Here's the drawing with two shaded views (mm, measured from the low corner). I have some questions. Give positions to 0.01 mm unless a question says otherwise; leave off trailing zeros. Loops run counter-clockwise (first coordinate to the right, second up) from the corner with the lowest first, then second, coordinate; pieces in that order, holes last.
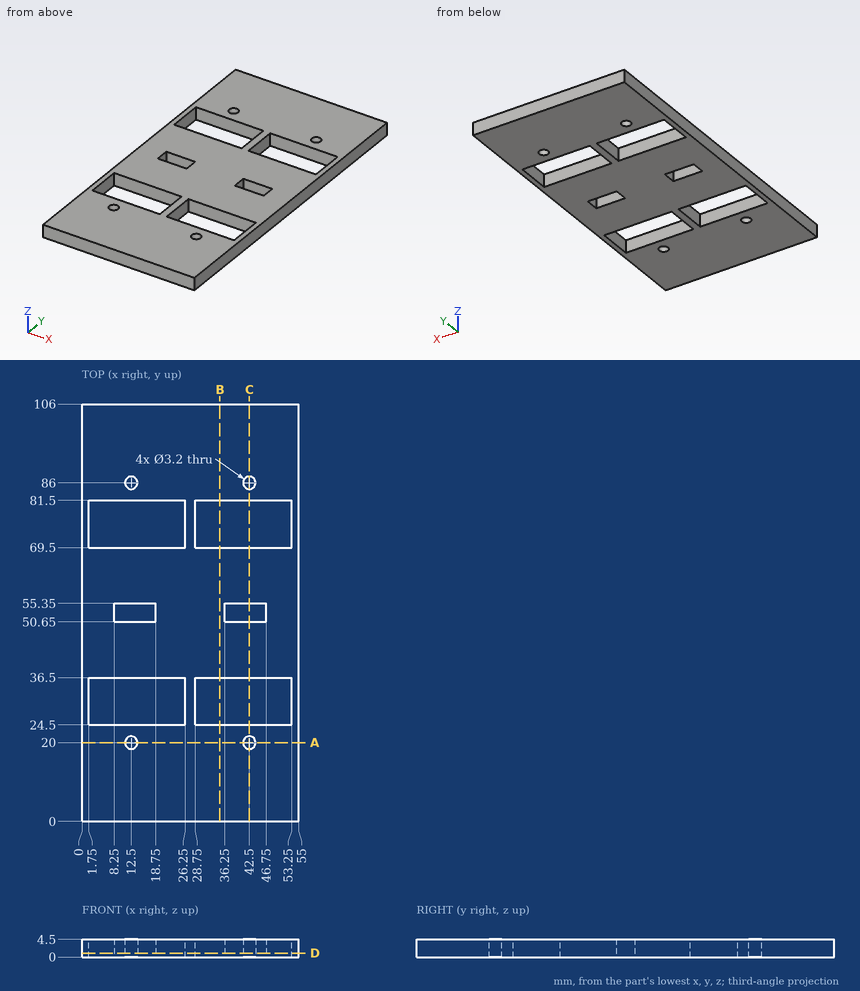
(1) Suppose I cut it at A-A on y = 20. List the corners of the cut face in (x, z) for me, plus the area to 3 significant figures.
Returned:
outline: (0, 0) - (10.9, 0) - (10.9, 4.5) - (0, 4.5) - close; (14.1, 0) - (40.9, 0) - (40.9, 4.5) - (14.1, 4.5) - close; (44.1, 0) - (55, 0) - (55, 4.5) - (44.1, 4.5) - close
area: 219 mm2
(2) Suppose I cut it at D-D on z = 1.05. Give the number of separate pieces and of enclosed holes in the cut face, plus the area to 3 significant figures.
Returned:
separate pieces: 1
enclosed holes: 10
area: 4,520 mm2
(3) Suppose I cut it at C-C on x = 42.5. List the corners of the cut face in (y, z) for me.
Returned:
outline: (0, 0) - (18.4, 0) - (18.4, 4.5) - (0, 4.5) - close; (21.6, 0) - (24.5, 0) - (24.5, 4.5) - (21.6, 4.5) - close; (36.5, 0) - (50.65, 0) - (50.65, 4.5) - (36.5, 4.5) - close; (55.35, 0) - (69.5, 0) - (69.5, 4.5) - (55.35, 4.5) - close; (81.5, 0) - (84.4, 0) - (84.4, 4.5) - (81.5, 4.5) - close; (87.6, 0) - (106, 0) - (106, 4.5) - (87.6, 4.5) - close
(4) Will these pins go through, and if not, where does the flat tip stop? P1, Ø1.9, axis at x = 12.5, y = 86, coming from the -Z side; P2, Ø1.3, axis at x = 17, z = 1.5, coming from the -Y side.
Returned:
P1: passes through
P2: stops at y = 0
(5) Suppose I cut it at B-B on x = 35. List the corners of the cut face in (y, z) for me.
Returned:
outline: (0, 0) - (24.5, 0) - (24.5, 4.5) - (0, 4.5) - close; (36.5, 0) - (69.5, 0) - (69.5, 4.5) - (36.5, 4.5) - close; (81.5, 0) - (106, 0) - (106, 4.5) - (81.5, 4.5) - close
(6) Please list where these lines run through material, in increasing order: probe 1 along Y at (x, z) = (42.5, 3.25); probe 2 along Y at (x, z) = (34, 0.7); probe 3 along Y at (x, z) = (9, 1.7).
Returned:
probe 1: y = 0 to 18.4, 21.6 to 24.5, 36.5 to 50.65, 55.35 to 69.5, 81.5 to 84.4, 87.6 to 106
probe 2: y = 0 to 24.5, 36.5 to 69.5, 81.5 to 106
probe 3: y = 0 to 24.5, 36.5 to 50.65, 55.35 to 69.5, 81.5 to 106
